Input: part model. Units: mm. Frame: model coordinates. Round coordinates to 2 decimals unless told otherwise and drop trailing zeros. Loops run counter-clockwise (first coordinate to the right, second up) from the corner with the lowest first, then second, coordinate; pieces in that order, holes last.
(1) Line query: line 1 (X direction, y = 0.5, z = 3.4); line 2 (X direction, y = -1.45, z = 1.7); line 3 (Y direction, x = 5, z = 1.6). Output: solid intervals per line, ascending.
(2) Cut plane B-B, the plane z = 3.4. Output: boundary loops of the cut face in (x, y), and give its area (3 significant figures).
(3) Draft query along X for faces 1 (the face through (-19.715, -2.699, 2.535)), 2 (the face through (3.35, 0.07, 2.54)), 3 (the face through (19.699, -2.715, 2.535)). Return one class per face: released by +X, released by -X, zero draft, split by the parting line, or undercut.
(4) Cut plane C-C, the plane y = 0. Output: boundary loops of the cut face in (x, z), and give its area (3 significant figures).
(5) Cut plane A-A, the plane x = 5. Output: boundary loops of the cut face in (y, z).
(6) First-contact query: pin 1 Ø3 at (x, y) = (5, 0) entering from +Z. Flat tip, straight axial feed; report the tip coordinate or a pass-through.
from build123d import *

# Parameters (mm, degrees)
SKETCH_1_W          = 40
SKETCH_1_H          = 6
EXTRUDE_1_DEPTH     = 5
SKETCH_2_R          = 1.65
CUT_EXTRUDE_1_DEPTH = 7
FILLET_1_R          = 1


with BuildPart() as part:
    # 草图1 → 凸台-拉伸1 (new body)
    with BuildSketch(Plane.XY):
        Rectangle(SKETCH_1_W, SKETCH_1_H)
    extrude(amount=EXTRUDE_1_DEPTH)

    # 草图2 → 切除-拉伸1 (cut)
    with BuildSketch(Plane.XY.offset(5)):
        with Locations((5, 0)):
            Circle(SKETCH_2_R)
        with Locations((-15, 0)):
            Circle(SKETCH_2_R)
    extrude(amount=-CUT_EXTRUDE_1_DEPTH, mode=Mode.SUBTRACT)

    # 圆角1
    fillet_1_edges = [part.edges().sort_by_distance(p)[0] for p in [
        (20, -3, 2.5),
        (-20, -3, 2.5),
        (-20, 3, 2.5),
        (20, 3, 2.5),
    ]]
    fillet(fillet_1_edges, radius=FILLET_1_R)


solid = part.part
Reported:
1. line 1: x = -20 to -16.57, -13.43 to 3.43, 6.57 to 20
1. line 2: x = -20 to -15.79, -14.21 to 4.21, 5.79 to 20
1. line 3: y = -3 to -1.65, 1.65 to 3
2. outline: (-20, -2) arc R1 ccw to (-19, -3) - (19, -3) arc R1 ccw to (20, -2) - (20, 2) arc R1 ccw to (19, 3) - (-19, 3) arc R1 ccw to (-20, 2) - close; hole circle Ø3.3 at (-15, 0); hole circle Ø3.3 at (5, 0)
2. area: 222 mm2
3. face 1: released by -X
3. face 2: undercut
3. face 3: released by +X
4. outline: (-20, 0) - (-16.65, 0) - (-16.65, 5) - (-20, 5) - close; (-13.35, 0) - (3.35, 0) - (3.35, 5) - (-13.35, 5) - close; (6.65, 0) - (20, 0) - (20, 5) - (6.65, 5) - close
4. area: 167 mm2
5. outline: (-3, 0) - (-1.65, 0) - (-1.65, 5) - (-3, 5) - close; (1.65, 0) - (3, 0) - (3, 5) - (1.65, 5) - close
6. pin 1: passes through
